The model under review builds one solid part; all positions refer to its coordinate system, in mm. Face numbers are marked on the shaded views. A direction names the side the tool comes from. Round coordinates to 2 decimals unless told otherwise and drop trailing zeros. Write each loop counter-clockwise with the first axis right and the second up, starting at its lowest first coordinate (ties: lowest second). Pieces come first, ordered by that corner, then holes. Notation, with made-up numbers: (31.25, 8) -> (82.25, 8) arc R18 cw to (82.25, 24) -> close; hole circle Ø2 at (49.25, 0). An arc over 180 degrees is marked (long way). Answer as a JSON object with one key per item and string values. Group by question number.
1) We need section D-D, the plane z = 5.75. Write out the cut boundary in (x, y).
2) Mouldability with a two-part tool opening along Y and no side actions: class the marked faces 1, 2 and 3 as pulls with the +Y half, pulls with the -Y half, needs draft (parallel to the pull), parting line crosses it, or undercut.
3) To check wall thickness, follow probe 1 along Y at (x, z) = (0, -1.4); probe 2 along Y at (x, z) = (0, 0.1). State the ranges of each line that lie inside material, in increasing order. Write a range as [from, to].
4) Machinability: for the marked faces 4 and 5, which of the approach directions +Z, -Z, +X, -X, +Y, -Y give a long, thin tool a straight path to every point of the face, cutting with its end or side? Answer none if there is none.
5) We need section C-C, the plane z = -0.25. Write out the cut boundary in (x, y).
6) We need section A-A, the plane y = 0. Write out the cut boundary in (x, z) (3 decimals).
7) Insertion check: pin 1 Ø4 at (x, z) = (3, 6.5) entering from -Y; pin 2 Ø2 at (x, z) = (-4.5, 7.5) entering from +Y; pin 3 Ø4 at (y, z) = (3.5, 8.5) entering from -X. Each pin has a flat end and moves straight along its axis. Give the tip position at first contact, or say it passes through.
from build123d import *

# Parameters (mm, degrees)
SKETCH_R     = 5.334
PAD_DEPTH    = 12.065
SKETCH001_R  = 7.003821
PAD001_DEPTH = 2.286
SKETCH002_R  = 4.572
POCKET_DEPTH = 3.302
FILLET_R     = 2.032


with BuildPart() as part:
    # Sketch → Pad (new body)
    with BuildSketch(Plane.XY):
        Circle(SKETCH_R)
    extrude(amount=PAD_DEPTH)

    # Sketch001 → Pad001 (new body)
    with BuildSketch(Plane(origin=(0, 0, 0), x_dir=(1, 0, 0), z_dir=(0, 0, -1))):
        Circle(SKETCH001_R)
    extrude(amount=PAD001_DEPTH)

    # Sketch002 → Pocket (cut)
    with BuildSketch(Plane(origin=(0, 0, -2.286), x_dir=(1, 0, 0), z_dir=(0, 0, -1))):
        Circle(SKETCH002_R)
    extrude(amount=-POCKET_DEPTH, mode=Mode.SUBTRACT)

    # Fillet
    fillet_edges = [part.edges().sort_by_distance(p)[0] for p in [
        (-5.334, 0, 12.065),
    ]]
    fillet(fillet_edges, radius=FILLET_R)


solid = part.part
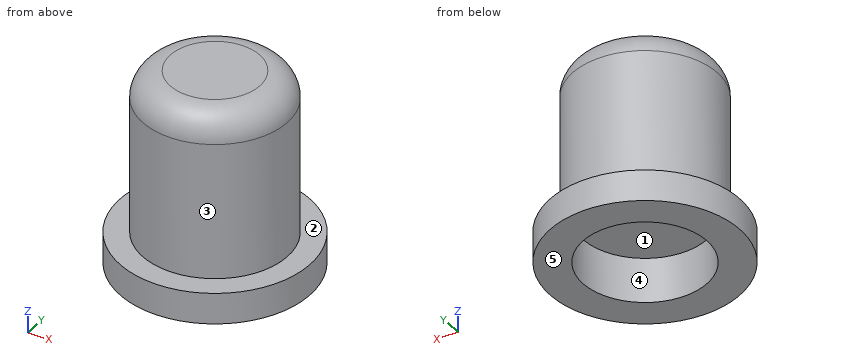
Here are the results:
{
 "1": {"outline": "circle Ø10.67 at (0, 0)"},
 "2": {"face 1": "undercut", "face 2": "needs draft", "face 3": "parting line crosses it"},
 "3": {"probe 1": "y = [-7, -4.57], [4.57, 7]", "probe 2": "y = [-5.33, -4.57], [4.57, 5.33]"},
 "4": {"face 4": "-Z", "face 5": "-Z, +X, -X, +Y, -Y"},
 "5": {"outline": "circle Ø14.01 at (0, 0); hole circle Ø9.14 at (0, 0)"},
 "6": {"outline": "(-7.004, -2.286) -> (-4.572, -2.286) -> (-4.572, 1.016) -> (4.572, 1.016) -> (4.572, -2.286) -> (7.004, -2.286) -> (7.004, 0) -> (5.334, 0) -> (5.334, 10.033) arc R2.032 ccw to (3.302, 12.065) -> (-3.302, 12.065) arc R2.032 ccw to (-5.334, 10.033) -> (-5.334, 0) -> (-7.004, 0) -> close"},
 "7": {"pin 1": "stops at y = -5.24", "pin 2": "stops at y = 4.03", "pin 3": "stops at x = -5.12"}
}
